Here's how the part is built. I have some questions about the finished solid (model axes, mm). A direction names the side the tool comes from. Round coordinates to 2 decimals unless told otherwise and drop trailing zeros. Order: outer loops, then holes, each group sorted by start corner. A loop starts at its lowest first (then second) coordinate and runs counter-clockwise, first axis right, second up. Notation, with made-up numbers: M 41,-30 L 89,-30 A26 ccw 89,-11 Z; hole C 74,87.5 d1. An arc over 180 degrees is marked long. Write item = value, one per line. Start each with the question number.
Item 1: I'm going to push flat-ended pins straight in: P1, Ø3, axis at x = -101.5, z = 148.5, coming from the -Y side; P2, Ø12, axis at x = -141, z = 108.5, coming from the +Y side; P3, Ø1, axis at x = -242, z = 87.5, coming from the +Y side. Where does each tip first touch, or does it pass through?
Item 2: I want a section at D-D, the plane y = 22.5. List the corners of the cut face in (x, z) for me, plus the area to 3 significant figures.
Item 3: I want a section at B-B, the plane x = -357. List the corners of the cut face in (y, z) for me.
Item 4: We'd pull the mould along Z, two halves only. Please class faces 3 (the face through (-338.022, 76.76, 50.862)), 4 (the face through (-387, 86, 176)), 5 (the face through (-193.21, 39.44, 88.74)): pulls with the +Z half, pulls with the -Z half, needs draft (parallel to the pull), parting line crosses it, or undercut.
Item 5: I want a section at C-C, the plane z = 119. List the corners of the cut face in (x, y) for me, plus the area to 3 significant figures.
Item 6: I want a section at A-A, the plane x = -305. List the corners of the cut face in (y, z) for me.
Item 7: Please list where these lines run through material, in increasing order: L1, parallel to Y at x = -158, z = 48; L2, parallel to Y at x = -149, z = 143.5.
Item 8: For faces 1 (the face through (-388.675, 87.1, 160.977)), 2 (the face through (-387, 86, 4)), which set-ups out of +Z, -Z, +X, -X, +Y, -Y let a thin tool reach every point of the face, with its end or its side?
```python
from build123d import *

# Parameters (mm, degrees)
BOSS_EXTRUDE3_DEPTH = 180
CUT_EXTRUDE1_DEPTH  = 180
FILLET1_R           = 13
FILLET2_R           = 13


with BuildPart() as part:
    # Sketch1 → Boss-Extrude3 (new body)
    with BuildSketch(Plane.XY):
        Polygon((0, 0), (-391.918358845, 80), (-388.918358845, 94.696938457), (3, 14.696938457), align=None)
    extrude(amount=BOSS_EXTRUDE3_DEPTH)

    # Sketch4 → Cut-Extrude1 (cut)
    with BuildSketch(Plane(origin=(3, 14.696938457, 0), x_dir=(0.9797958971132712, -0.2, 0), z_dir=(0.2, 0.9797958971132712, 0))):
        Polygon((-400, -20), (-278.75644347, -90), (-400, -160), align=None)
    extrude(amount=-CUT_EXTRUDE1_DEPTH, mode=Mode.SUBTRACT)

    # Fillet1
    # the kernel refuses this fillet: 13 mm, written as the material it takes off along each edge
    with BuildSketch(Plane(origin=(-398.418358845, 48.156633344, 0), x_dir=(0.9797958971132713, -0.19999999999999976, 0), z_dir=(0.19999999999999976, 0.9797958971132713, 0)), Plane(origin=(-398.418358845, 48.156633344, 180), x_dir=(0, 0, -1), z_dir=(0.19999999999999976, 0.9797958971132713, 0))) as fillet1_piece_1:
        with BuildLine():
            CenterArc((FILLET1_R, -FILLET1_R), FILLET1_R, 90, 90)
            Line((0, -FILLET1_R), (0, 0))
            Line((0, 0), (FILLET1_R, 0))
        make_face()
    extrude(amount=80, mode=Mode.SUBTRACT)
    with BuildSketch(Plane(origin=(-385.165582096, 113.081714768, 20), x_dir=(0, 0, -1), z_dir=(-0.20000000000000004, -0.9797958971132713, 0)), Plane(origin=(-385.165582096, 113.081714768, 160), x_dir=(0.8485281374238575, -0.17320508075688784, -0.4999999999999992), z_dir=(-0.20000000000000004, -0.9797958971132713, 0))) as fillet1_piece_2:
        with BuildLine():
            CenterArc((FILLET1_R * 0.57735026919, FILLET1_R), FILLET1_R, 210, 60)
            Line((-FILLET1_R * 0.288675134595, FILLET1_R * 0.5), (0, 0))
            Line((0, 0), (FILLET1_R * 0.57735026919, 0))
        make_face()
    extrude(amount=52.527767497, mode=Mode.SUBTRACT)

    # Fillet2
    fillet2_edges = [part.edges().sort_by_distance(p)[0] for p in [
        (-271.624419606, 63.099757922, 90),
    ]]
    fillet(fillet2_edges, radius=FILLET2_R)


solid = part.part
```
Filled in:
q1.P1 = 20.41
q1.P2 = 45.32
q1.P3 = 64.81
q2.outline = M -110.23,0 L -35.23,0 L -35.23,180 L -110.23,180 Z
q2.area = 13,500 mm^2
q3.outline = M 72.87,0 L 88.18,0 L 88.18,38.81 L 72.87,40.58 Z; M 72.87,139.42 L 88.18,141.19 L 88.18,180 L 72.87,180 Z
q4.face_3 = undercut
q4.face_4 = pulls with the +Z half
q4.face_5 = needs draft
q5.outline = M -322.34,65.8 L 0,0 L 3,14.7 L -319.34,80.49 Z
q5.area = 4,930 mm^2
q6.outline = M 62.26,0 L 77.57,0 L 77.57,69.45 L 62.26,71.22 Z; M 62.26,108.78 L 77.57,110.55 L 77.57,180 L 62.26,180 Z
q7.L1 = 32.25 to 47.56
q7.L2 = 30.41 to 45.72
q8.face_1 = -X, +Y
q8.face_2 = -Z, -X, +Y
